CAD build for the part. Positions are in the model's coordinates, mm. A direction names the side the tool comes from. Round coordinates to 2 decimals unless told otherwise and drop trailing zeros. Loops run counter-clockwise (first coordinate to the right, second up) from the corner with the lowest first, then second, coordinate; pieces in that order, holes last. Notation, with made-up numbers: M 55.5,60 L 106.5,60 A37 cw 106.5,97 Z; hole C -24.75,-15.5 d6. An arc over 180 degrees is marked long. Put each result on its own line as item: value. Start each with the question number.
from build123d import *

# Parameters (mm, degrees)
SKETCH1_W           = 25.6
SKETCH1_H           = 44.7
BOSS_EXTRUDE1_DEPTH = 16.8
FILLET1_R           = 2
BOSS_EXTRUDE2_START = -44.7
SKETCH2_R           = 2.75
BOSS_EXTRUDE2_DEPTH = 47.3
CUT_EXTRUDE1_DEPTH  = 0.1


with BuildPart() as part:
    # Sketch1 → Boss-Extrude1 (new body)
    with BuildSketch(Plane(origin=(0, 0, 0), x_dir=(1, 0, 0), z_dir=(0, 1, 0))):
        with Locations((-11.517488789, 20.134753363)):
            Rectangle(SKETCH1_W, SKETCH1_H)
    extrude(amount=BOSS_EXTRUDE1_DEPTH)

    # Fillet1
    fillet1_edges = [part.edges().sort_by_distance(p)[0] for p in [
        (1.282511211, 16.8, -20.134753363),
        (-24.317488789, 16.8, -20.134753363),
        (1.282511211, 0, -20.134753363),
        (-24.317488789, 0, -20.134753363),
    ]]
    fillet(fillet1_edges, radius=FILLET1_R)

    # Sketch2 → Boss-Extrude2 (add)
    with BuildSketch(Plane(origin=(0, 0, -42.484753363), x_dir=(-1, 0, 0), z_dir=(0, 0, -1)).offset(BOSS_EXTRUDE2_START)):
        with Locations((17.767488789, 8.4)):
            Circle(SKETCH2_R)
        Polygon((5.067488789, 12.730127019), (1.317488789, 10.565063509), (1.317488789, 6.234936491), (5.067488789, 4.069872981), (8.817488789, 6.234936491), (8.817488789, 10.565063509), align=None)
    extrude(amount=BOSS_EXTRUDE2_DEPTH)

    # Sketch3 → Cut-Extrude1 (cut)
    # profile 1 of 2: a face of its own
    with BuildSketch(Plane(origin=(0, 16.8, 0), x_dir=(1, 0, 0), z_dir=(0, 1, 0))):
        with BuildLine():
            Line((-13.318041778, 18.082325539), (-13.569043381, 18.256904866))
            Line((-13.569043381, 18.256904866), (-12.595886329, 19.679480988))
            add(Edge.make_bspline(
                [(-12.595886329, 19.679480988), (-12.657977065, 19.671887924), (-12.780237185, 19.656936759), (-12.903374287, 19.654190105), (-12.963975272, 19.652838359)],
                knots=[0, 0, 0, 0, 1.015715272, 2, 2, 2, 2], degree=3))
            add(Edge.make_bspline(
                [(-12.963975272, 19.652838359), (-13.00071732, 19.653779436), (-13.072838746, 19.655626687), (-13.178870399, 19.670268495), (-13.280755959, 19.692818623), (-13.378225315, 19.726467378), (-13.47164482, 19.768285587), (-13.560810534, 19.8201426), (-13.645602424, 19.881148892), (-13.725109834, 19.950981884), (-13.797421573, 20.027659936), (-13.861844871, 20.108815579), (-13.915386003, 20.19539155), (-13.959862588, 20.285621769), (-13.993593042, 20.38080312), (-14.018155579, 20.47985252), (-14.033277934, 20.583464162), (-14.035077029, 20.653989293), (-14.035990496, 20.689797494)],
                knots=[0, 0, 0, 0, 1.060718605, 2.082097864, 3.085795603, 4.069760067, 5.054557537, 6.03741023, 7.043284206, 8.066802108, 9.088538119, 10.083643548, 11.053783639, 12.022749082, 12.983451788, 13.964007469, 14.966251758, 16, 16, 16, 16], degree=3))
            add(Edge.make_bspline(
                [(-14.035990496, 20.689797494), (-14.034256061, 20.738766147), (-14.030851718, 20.834881678), (-14.0034532, 20.975315447), (-13.958392861, 21.108101991), (-13.895564484, 21.232892185), (-13.816429763, 21.347890924), (-13.721321173, 21.451499533), (-13.610817209, 21.542244387), (-13.487435189, 21.620248464), (-13.354082169, 21.682983462), (-13.214413511, 21.729222762), (-13.069499391, 21.75642151), (-12.97133172, 21.760007371), (-12.921907964, 21.761812718)],
                knots=[0, 0, 0, 0, 1.022988612, 2.007919123, 2.978103895, 3.94594894, 4.918897164, 5.887013414, 6.875921846, 7.89917871, 8.930658928, 9.948724884, 10.967259574, 12, 12, 12, 12], degree=3))
            add(Edge.make_bspline(
                [(-12.921907964, 21.761812718), (-12.873419544, 21.759982555), (-12.777610998, 21.756366326), (-12.636721991, 21.729882357), (-12.501780974, 21.685245684), (-12.373535987, 21.62356112), (-12.254796575, 21.546240212), (-12.148020764, 21.454105689), (-12.055645225, 21.347100161), (-11.977821344, 21.227811671), (-11.915351304, 21.09964469), (-11.870279021, 20.965860768), (-11.842533382, 20.827422046), (-11.839037055, 20.733627572), (-11.837272547, 20.686291885)],
                knots=[0, 0, 0, 0, 1.026385292, 2.028040595, 3.023318987, 4.028184125, 5.03290303, 6.015178782, 7.004435299, 8.016004309, 9.023023918, 10.015172535, 10.998308025, 12, 12, 12, 12], degree=3))
            add(Edge.make_bspline(
                [(-11.837272547, 20.686291885), (-11.838450956, 20.649548118), (-11.840841064, 20.575022577), (-11.857577371, 20.461792234), (-11.885997556, 20.346341005), (-11.918249255, 20.248619409), (-11.949381423, 20.167910959), (-11.978682554, 20.104159379), (-12.011194708, 20.037058116), (-12.049113473, 19.967310778), (-12.08987577, 19.894028243), (-12.135935047, 19.817945527), (-12.186240619, 19.738960534), (-12.222070338, 19.685713446), (-12.240417579, 19.658447334)],
                knots=[0, 0, 0, 0, 1.179839688, 2.393009684, 3.667231171, 4.993948276, 5.694988576, 6.444077775, 7.246288328, 8.089075292, 8.993003841, 9.939041771, 10.944649915, 12, 12, 12, 12], degree=3))
            Line((-12.240417579, 19.658447334), (-13.318041778, 18.082325539))
        make_face()
        with BuildLine():
            add(Edge.make_bspline(
                [(-12.905782163, 20.011812718), (-12.877948149, 20.012573102), (-12.823764786, 20.014053311), (-12.744387487, 20.023062553), (-12.669463283, 20.039036539), (-12.598792034, 20.061956251), (-12.531665132, 20.08961292), (-12.469148804, 20.124824906), (-12.411190728, 20.166841541), (-12.357402801, 20.214051556), (-12.309638802, 20.26650214), (-12.267095771, 20.321399247), (-12.230935204, 20.378983857), (-12.202371926, 20.439977119), (-12.178887351, 20.502894327), (-12.162669339, 20.568748683), (-12.153685006, 20.637197083), (-12.152153431, 20.683695741), (-12.151375111, 20.707325539)],
                knots=[0, 0, 0, 0, 1.163407946, 2.26475976, 3.333800367, 4.359385343, 5.366239384, 6.363380779, 7.350133999, 8.353570782, 9.349036268, 10.310270964, 11.253520213, 12.184142, 13.120487599, 14.056272588, 15.012232024, 16, 16, 16, 16], degree=3))
            add(Edge.make_bspline(
                [(-12.151375111, 20.707325539), (-12.152044781, 20.730965204), (-12.153364446, 20.777550064), (-12.163951746, 20.846099804), (-12.182576969, 20.911793065), (-12.207567453, 20.974989495), (-12.240487691, 21.035169867), (-12.279991177, 21.093089738), (-12.326923627, 21.148381866), (-12.380926193, 21.19974585), (-12.439160746, 21.247093749), (-12.501221246, 21.288879825), (-12.566596162, 21.323901021), (-12.634886652, 21.352799991), (-12.706235001, 21.375351767), (-12.780598989, 21.391569132), (-12.858354395, 21.400540886), (-12.911135681, 21.402062781), (-12.938033765, 21.402838359)],
                knots=[0, 0, 0, 0, 0.972161553, 1.915763587, 2.844109794, 3.775983486, 4.705125789, 5.659731448, 6.655561913, 7.682237399, 8.721216875, 9.739758359, 10.754845918, 11.767244016, 12.7857855, 13.828538656, 14.893392813, 16, 16, 16, 16], degree=3))
            add(Edge.make_bspline(
                [(-12.938033765, 21.402838359), (-12.964697919, 21.402061528), (-13.017012768, 21.40053739), (-13.094076927, 21.391586185), (-13.167938095, 21.375242701), (-13.239079716, 21.352810437), (-13.307368176, 21.323898866), (-13.372740009, 21.28887799), (-13.434815026, 21.247103368), (-13.492993746, 21.199708595), (-13.547091668, 21.148620949), (-13.593217197, 21.09284752), (-13.63281109, 21.035199996), (-13.665686092, 20.974981487), (-13.69068861, 20.911795202), (-13.709310611, 20.846099225), (-13.719898776, 20.777550215), (-13.721218323, 20.730965255), (-13.721887932, 20.707325539)],
                knots=[0, 0, 0, 0, 1.099389452, 2.15699305, 3.192601482, 4.213358962, 5.227959689, 6.245255729, 7.266013209, 8.307253147, 9.336162325, 10.327954924, 11.284637477, 12.215801273, 13.149702402, 14.080068371, 15.025723358, 16, 16, 16, 16], degree=3))
            add(Edge.make_bspline(
                [(-13.721887932, 20.707325539), (-13.721282006, 20.68367734), (-13.720087009, 20.637038764), (-13.708559219, 20.568512371), (-13.689280939, 20.502824177), (-13.663461549, 20.43933547), (-13.629459958, 20.378663612), (-13.58773611, 20.32109625), (-13.538830564, 20.2659808), (-13.483397077, 20.214173588), (-13.422728916, 20.166621412), (-13.35793217, 20.12509103), (-13.290122333, 20.090018586), (-13.219060702, 20.061877202), (-13.145273902, 20.039265539), (-13.068098771, 20.023091993), (-12.987790533, 20.014139727), (-12.933380551, 20.01259583), (-12.905782163, 20.011812718)],
                knots=[0, 0, 0, 0, 0.952633368, 1.87876736, 2.791047057, 3.707742249, 4.635551637, 5.587206343, 6.568248508, 7.601284464, 8.641511608, 9.671105535, 10.699146789, 11.713763218, 12.747829548, 13.806491675, 14.887386225, 16, 16, 16, 16], degree=3))
        make_face(mode=Mode.SUBTRACT)
    # profile 2 of 2: a face of its own
    with BuildSketch(Plane(origin=(0, 16.8, 0), x_dir=(1, 0, 0), z_dir=(0, 1, 0))):
        Polygon((-11.343682804, 21.672069129), (-11.007144342, 21.672069129), (-9.840477676, 18.913855988), (-8.673811009, 21.672069129), (-8.337272547, 21.672069129), (-9.818041778, 18.172069129), (-9.862913573, 18.172069129), align=None)
    extrude(amount=-CUT_EXTRUDE1_DEPTH, mode=Mode.SUBTRACT)


solid = part.part
(1) Flat gauge pin, fed straight in: pin 1 Ø3 at (y, z) = (9.5, -43.5) entering from -X. Where does the tip first touch, or does it go through?
(2) Cut at B-B on x = -3. List the corners of the cut face in (y, z).
(3) Cut at D-D on x = -21. List the corners of the cut face in (y, z), and give its area (3 significant figures).
(4) Cut at A-A on y = 8.4. List the corners of the cut face in (x, z).
(5) Cut at C-C on y = 12.25. List the corners of the cut face in (x, z), and give its area (3 significant figures).
(6) Drill centre lines: line 1 along Z through (x, y) = (-5, 1); line 2 along Y through (x, z) = (-0.5, -35.5); line 3 along X through (y, z) = (15.25, -23.5). Where is each one in solid material? Low to high.
(7) Mould opens along X. For faces 1 (the flat face through (-5, 8, -45.085)), 2 (the flat face through (-24.317, 8, -20)), 3 (the flat face through (-6.97, 11.63, -43.77)), 4 (the flat face through (1.283, 8, -20)) say: +X half, -X half, draft (parallel to the pull), parting line (faces both ways), or undercut.
(8) Tool access for faces 5 (the flat face through (-6.92, 5.14, -43.77)), 6 (the cylindrical face through (-17.171, 5.715, -43.767)), 7 (the cylindrical face through (0.71, 16.2, -20.45)): list every direction of +Z, -Z, +X, -X, +Y, -Y with a clear straight run to the whole face (end or side of a thin tool).
Taken from the geometry:
1. pin 1: x = -24.32
2. outline: M 0,-42.48 L 5.26,-42.48 L 5.26,-45.08 L 11.54,-45.08 L 11.54,-42.48 L 16.8,-42.48 L 16.8,2.22 L 0,2.22 Z
3. outline: M 0,-42.48 L 16.8,-42.48 L 16.8,2.22 L 0,2.22 Z
3. area: 751 mm2
4. outline: M -24.32,-42.48 L -20.52,-42.48 L -20.52,-45.08 L -15.02,-45.08 L -15.02,-42.48 L -8.82,-42.48 L -8.82,-45.08 L -1.32,-45.08 L -1.32,-42.48 L 1.28,-42.48 L 1.28,2.22 L -24.32,2.22 Z
5. outline: M -24.32,-42.48 L -5.9,-42.48 L -5.9,-45.08 L -4.24,-45.08 L -4.24,-42.48 L 1.28,-42.48 L 1.28,2.22 L -24.32,2.22 Z
5. area: 1,150 mm2
6. line 1: -42.48 to 2.22
6. line 2: 0.01 to 16.79
6. line 3: -24.27 to 1.23
7. face 1: draft
7. face 2: -X half
7. face 3: undercut
7. face 4: +X half
8. face 5: -Z, -Y
8. face 6: -Z
8. face 7: +Z, -Z, +X, +Y
